Here's how the part is built. I have some questions about the finished solid (model axes, mm). A direction names the side the tool comes from. Round coordinates to 2 decimals unless told otherwise and drop trailing zeros. Write each loop counter-clockwise with the first axis right and the second up, starting at its lowest first coordinate (ties: lowest second). Pieces come first, ordered by that corner, then holes. Notation, with made-up numbers: (34, 34.5) - (71, 34.5) arc R19 cw to (71, 47.5) - close; hole circle Ø6 at (69.25, 34). An arc over 180 degrees is marked (long way). Return JSON: item names as keys, results as strings. Group by question number.
```python
from build123d import *

# Parameters (mm, degrees)
SKETCH1_W           = 5
SKETCH1_H           = 5
BOSS_EXTRUDE1_DEPTH = 5


with BuildPart() as part:
    # Sketch1 → Boss-Extrude1 (new body)
    with BuildSketch(Plane.XY):
        with BuildLine():
            Line((17.5, -5), (10.481741735, -5))
            ThreePointArc((10.481741735, -5), (8.951008006, -5.30448187), (7.653314611, -6.171572875))
            Line((7.653314611, -6.171572875), (6.171572875, -7.653314611))
            ThreePointArc((6.171572875, -7.653314611), (5.30448187, -8.951008006), (5, -10.481741735))
            Line((5, -10.481741735), (5, -17.5))
            Line((5, -17.5), (5, -22.5))
            Line((5, -22.5), (5, -26))
            Line((5, -26), (8, -26))
            Line((8, -26), (8, -24.9))
            Line((8, -24.9), (10.3, -24.9))
            Line((10.3, -24.9), (10.3, -26))
            Line((10.3, -26), (15, -26))
            Line((15, -26), (15, -29))
            Line((15, -29), (10.3, -29))
            Line((10.3, -29), (10.3, -30.1))
            Line((10.3, -30.1), (8, -30.1))
            Line((8, -30.1), (8, -29))
            Line((8, -29), (5, -29))
            Line((5, -29), (5, -32.5))
            Line((5, -32.5), (5, -37.5))
            Line((5, -37.5), (5, -43.5))
            ThreePointArc((5, -43.5), (6.171572875, -46.328427125), (9, -47.5))
            Line((9, -47.5), (9.165507919, -47.5))
            ThreePointArc((9.165507919, -47.5), (10.696241649, -47.19551813), (11.993935044, -46.328427125))
            Line((11.993935044, -46.328427125), (46.328427125, -11.993935044))
            ThreePointArc((46.328427125, -11.993935044), (47.19551813, -10.696241649), (47.5, -9.165507919))
            Line((47.5, -9.165507919), (47.5, -9))
            ThreePointArc((47.5, -9), (46.328427125, -6.171572875), (43.5, -5))
            Line((43.5, -5), (37.5, -5))
            Line((37.5, -5), (32.5, -5))
            Line((32.5, -5), (29, -5))
            Line((29, -5), (29, -8))
            Line((29, -8), (30.1, -8))
            Line((30.1, -8), (30.1, -10.3))
            Line((30.1, -10.3), (29, -10.3))
            Line((29, -10.3), (29, -15))
            Line((29, -15), (26, -15))
            Line((26, -15), (26, -10.3))
            Line((26, -10.3), (24.9, -10.3))
            Line((24.9, -10.3), (24.9, -8))
            Line((24.9, -8), (26, -8))
            Line((26, -8), (26, -5))
            Line((26, -5), (22.5, -5))
            Line((22.5, -5), (17.5, -5))
        make_face()
        with Locations((2.5, -20)):
            Rectangle(SKETCH1_W, SKETCH1_H)
        with Locations((20, -2.5)):
            Rectangle(SKETCH1_W, SKETCH1_H)
        with Locations((35, -2.5)):
            Rectangle(SKETCH1_W, SKETCH1_H)
        with Locations((2.5, -35)):
            Rectangle(SKETCH1_W, SKETCH1_H)
    extrude(amount=BOSS_EXTRUDE1_DEPTH)


solid = part.part
```
1) Will these pins go through, and if not, where does the flat tip stop? pin 1 Ø1.5 at (y, z) = (-23.5, 4) entering from +X; pin 2 Ø2 at (x, z) = (31.5, 2) entering from -Y; pin 3 Ø1.5 at (y, z) = (-40.5, 2) entering from -X.
2) Imagine slicing it at B-B (y = -42.5). Please give me the cut outline in (x, z).
3) Imagine slicing it at A-A (x = 3). Please give me the cut outline in (y, z), plus the area to 3 significant figures.
4) If we mould it in two halves opening along Y, with no side actions, what happens to faces 4 (the flat face through (25.5, -10.3, 2.5)), 5 (the cylindrical face through (6.141, -46.297, 2.465)), 6 (the flat face through (29, -13, 2))? For each: released by +Y, released by -Y, zero draft, split by the parting line, or undercut.
5) Imagine slicing it at C-C (x = 38.5). Please give me the cut outline in (y, z).
6) For faces 1 (the flat face through (13, -29, 2)), 2 (the flat face through (2, -17.5, 2)), 3 (the flat face through (29, -6, 2)), which set-ups out of +Z, -Z, +X, -X, +Y, -Y let a thin tool reach every point of the face, with its end or its side?
7) I need wall thicknesses on line 1 along Y through (x, z) = (4, 0.8); line 2 along X through (y, z) = (-14, 1.75); line 3 along X through (y, z) = (-25, 2.45). Which ranges of each line are inside material? Lowest first, please.
Results found:
{
 "1": {"pin 1": "stops at x = 35.57", "pin 2": "stops at y = -27.82", "pin 3": "stops at x = 5"},
 "2": {"outline": "(5, 0) - (15.82, 0) - (15.82, 5) - (5, 5) - close"},
 "3": {"outline": "(-37.5, 0) - (-32.5, 0) - (-32.5, 5) - (-37.5, 5) - close; (-22.5, 0) - (-17.5, 0) - (-17.5, 5) - (-22.5, 5) - close", "area": "50.0 mm²"},
 "4": {"face 4": "undercut", "face 5": "released by -Y", "face 6": "zero draft"},
 "5": {"outline": "(-19.82, 0) - (-5, 0) - (-5, 5) - (-19.82, 5) - close"},
 "6": {"face 1": "+Z, -Z, -X", "face 2": "+Z, -Z, -X, +Y", "face 3": "+Z, -Z, +Y"},
 "7": {"line 1": "y = -37.5 to -32.5, -22.5 to -17.5", "line 2": "x = 5 to 26, 29 to 44.32", "line 3": "x = 5 to 8, 10.3 to 33.32"}
}
